from build123d import *

# Parameters (mm, degrees)
EXTRUDE_1_DEPTH          = 28.5
FILLET_3_R               = 4
CUT_EXTRUDE_1_DEPTH      = 31.686479107
CUT_EXTRUDE_1_DEPTH_BACK = 31.686479107
SKETCH_4_W               = 15
SKETCH_4_H               = 29
CUT_EXTRUDE_5_DEPTH      = 1.2
CUT_EXTRUDE_6_DEPTH      = 5
CUT_EXTRUDE_6_DEPTH_BACK = 25
SKETCH_5_R               = 2.6
CUT_EXTRUDE_7_DEPTH      = 31.823043328
DRAFT_1_ANGLE            = 60
SKETCH_7_W               = 10
SKETCH_7_H               = 1.2
SKETCH_7_H_2             = 0.5
CUT_EXTRUDE_8_DEPTH      = 31.686479107
DRAFT_3_ANGLE            = 30
SKETCH_8_W               = 17
SKETCH_8_H               = 30
CUT_EXTRUDE_9_DEPTH      = 2


with BuildPart() as part:
    # Эскиз2 → Бобышка-Вытянуть1 (new, symmetric)
    with BuildSketch(Plane.XY):
        Polygon((-10, 1.5), (-3, 2.9), (0, 2.9), (3, 2.9), (10, 1.5), (11, 1.5), (11, -1.5), (10, -1.5), (3, -2.9), (0, -2.9), (-3, -2.9), (-10, -1.5), (-11, -1.5), (-11, 1.5), align=None)
    extrude(amount=EXTRUDE_1_DEPTH, both=True)

    # Скругление3
    fillet_3_edges = [part.edges().sort_by_distance(p)[0] for p in [
        (-11, 0, -28.5),
        (-11, 0, 28.5),
        (11, 0, 28.5),
        (11, 0, -28.5),
    ]]
    fillet(fillet_3_edges, radius=FILLET_3_R)

    # Эскиз3 → Вырез-Вытянуть1 (cut, two sides: drawn at the far end of the back side and taken through both)
    with BuildSketch(Plane(origin=(0, 0, 0), x_dir=(0, 0, -1), z_dir=(1, 0, 0)).offset(-CUT_EXTRUDE_1_DEPTH_BACK)):
        Polygon((28.5, 2.9), (25.5, 2.9), (27.5, 1.5), (28.5, 1.5), align=None)
        Polygon((-27.5, -1.5), (-28.5, -1.5), (-28.5, -2.9), (-25.5, -2.9), align=None)
        Polygon((-25.5, 2.9), (-28.5, 2.9), (-28.5, 1.5), (-27.5, 1.5), align=None)
        Polygon((25.5, -2.9), (28.5, -2.9), (28.5, -1.5), (27.5, -1.5), align=None)
    extrude(amount=CUT_EXTRUDE_1_DEPTH + CUT_EXTRUDE_1_DEPTH_BACK, mode=Mode.SUBTRACT)

    # Эскиз4 → Вырез-Вытянуть5 (cut, symmetric)
    with BuildSketch(Plane(origin=(0, 0, 0), x_dir=(1, 0, 0), z_dir=(0, 1, 0))):
        with Locations((0, -12)):
            Rectangle(SKETCH_4_W, SKETCH_4_H)
    extrude(amount=CUT_EXTRUDE_5_DEPTH, both=True, mode=Mode.SUBTRACT)

    # Эскиз5 → Вырез-Вытянуть6 (cut, two sides: drawn at the far end of the back side and taken through both)
    with BuildSketch(Plane.XY.offset(-2.5).offset(-CUT_EXTRUDE_6_DEPTH_BACK)):
        with Locations(Location((0, 0, 0), (0, 0, 152.51357375))):
            Circle(SKETCH_5_R)
    extrude(amount=CUT_EXTRUDE_6_DEPTH + CUT_EXTRUDE_6_DEPTH_BACK, mode=Mode.SUBTRACT)

    # Эскиз6 → Вырез-Вытянуть7 (cut, through all)
    with BuildSketch(Plane.XZ.offset(-1.2)):
        Polygon((-2.306512519, -2.5), (2.306512519, -2.5), (7.5, -2.5), (7.5, 26.5), (-7.5, 26.5), (-7.5, -2.5), align=None)
    extrude(amount=-CUT_EXTRUDE_7_DEPTH, mode=Mode.SUBTRACT)

    # Уклон1
    draft_1_faces = [part.faces().sort_by_distance(p)[0] for p in [
        (0, -1.775343229, 2.5),
    ]]
    draft(draft_1_faces, Plane.ZX.offset(-1.2), DRAFT_1_ANGLE)

    # Эскиз7 → Вырез-Вытянуть8 (cut, through all)
    with BuildSketch(Plane(origin=(0, 0, 0), x_dir=(0, 0, -1), z_dir=(1, 0, 0))):
        with Locations((-13.5, -0.6)):
            Rectangle(SKETCH_7_W, SKETCH_7_H)
        with Locations((-13.5, -1.45)):
            Rectangle(SKETCH_7_W, SKETCH_7_H_2)
    extrude(amount=CUT_EXTRUDE_8_DEPTH, mode=Mode.SUBTRACT)

    # Уклон3
    draft_3_faces = [part.faces().sort_by_distance(p)[0] for p in [
        (0, -1.45, 13.5),
    ]]
    draft(draft_3_faces, Plane(origin=(11, 0, 18.5), x_dir=(-1, 0, 0), z_dir=(0, 0, -1)), DRAFT_3_ANGLE)

    # Эскиз8 → Вырез-Вытянуть9 (cut)
    with BuildSketch(Plane(origin=(0, 2.9, 0), x_dir=(1, 0, 0), z_dir=(0, 1, 0))):
        with Locations((0, -11.5)):
            Rectangle(SKETCH_8_W, SKETCH_8_H)
    extrude(amount=-CUT_EXTRUDE_9_DEPTH, mode=Mode.SUBTRACT)


solid = part.part
Work out the finished part from the listing and answer in its coordinate system (mm). A direction names the side the tool comes from. Round coordinates to 2 decimals unless told otherwise and drop trailing zeros. Write each loop counter-clockwise with the first axis right and the second up, starting at its lowest first coordinate (ties: lowest second). Pieces come first, ordered by that corner, then holes. Notation, with made-up numbers: (37.5, -2) -> (45.5, -2) arc R14 cw to (45.5, 4) -> close; hole circle Ø8 at (23.5, 52.5). An arc over 180 degrees is marked (long way). Write each question's results on one line, items separated by ' | '.
Item 1: Flat-ended cylindrical pins translate along their axes: P1, Ø0.5, axis at x = -4.5, z = -28, coming from the -Y side; P2, Ø1.1, axis at x = -1, z = -28, coming from the +Y side; P3, Ø1.8, axis at x = 9.5, z = 11.5, coming from the -Y side. Find the tip coordinate at first contact, or state that the pin passes through.
Result set:
P1: y = -1.5 | P2: y = 1.5 | P3: y = -1.78
Item 2: A cutting plane is placed at A-A, the plane z = -24. Determine the outline of the cut face in (x, y), plus the area to 3 significant figures.
Result set:
outline: (-11, -1.5) -> (-10, -1.5) -> (-3, -2.9) -> (3, -2.9) -> (10, -1.5) -> (11, -1.5) -> (11, 1.5) -> (10, 1.5) -> (3, 2.9) -> (-3, 2.9) -> (-10, 1.5) -> (-11, 1.5) -> close; hole circle Ø5.2 at (0, 0) | area: 81.2 mm^2
Item 3: Which of the six approach directions +Z, -Z, +X, -X, +Y, -Y give full straight-line access (tool end or side, diameter ignored) to faces 1 (the face through (-5, 0, -2.5)), 2 (the face through (6.6, -1.4, 18.5)), 3 (the face through (0, 0, -27.5))?
Result set:
face 1: +Y | face 2: +X | face 3: none
Item 4: Find the intervals of material crossed by line 1 along X through (y, z) = (0, -16); line 2 along Z through (x, y) = (-7.25, 0.3); line 3 along Y through (x, z) = (-0.25, -19), in increasing order. Write a range as [from, to].
Result set:
line 1: [-11, -2.6], [2.6, 11] | line 2: [-28.49, -2.5], [26.5, 28.49] | line 3: [-2.9, -2.59], [2.59, 2.9]
Item 5: A cutting plane is placed at B-B, the plane x = 1.25. Determine the outline of the cut face in (y, z), plus the area to 3 significant figures.
Result set:
outline: (-2.9, -25.5) -> (-2.28, -26.39) -> (-2.28, 0.63) -> (-1.2, 2.5) -> (-1.2, 8.5) -> (-1.7, 8.5) -> (-1.7, 18.5) -> (-1.2, 18.5) -> (-1.2, 26.5) -> (2.2, 26.5) -> (1.5, 27.5) -> (1.5, 28.5) -> (-1.5, 28.5) -> (-1.5, 27.5) -> (-2.9, 25.5) -> close; (-1.5, -28.5) -> (1.5, -28.5) -> (1.5, -27.5) -> (-1.5, -27.5) -> close; (2.28, -26.39) -> (2.9, -25.5) -> (2.9, -3.5) -> (2.28, -3.5) -> close | area: 77.7 mm^2
Item 6: The mould has two halves that part along Z. Classify faces 4 (the face through (7.5, 0.3, 11.8)), 5 (the face through (0, 0, -28.5)), 6 (the face through (0, -1.5, -28)): +Z half, -Z half, draft (parallel to the pull), parting line (faces both ways), or undercut.
Result set:
face 4: undercut | face 5: -Z half | face 6: draft
Item 7: A cutting plane is placed at D-D, the plane y = -0.65. Determine the outline of the cut face in (x, z).
Result set:
outline: (-11, -24.5) arc R4 ccw to (-7, -28.5) -> (7, -28.5) arc R4 ccw to (11, -24.5) -> (11, 8.5) -> (7.5, 8.5) -> (7.5, -2.5) -> (2.52, -2.5) -> (2.52, -27.5) -> (-2.52, -27.5) -> (-2.52, -2.5) -> (-7.5, -2.5) -> (-7.5, 26.5) -> (7.5, 26.5) -> (7.5, 18.5) -> (11, 18.5) -> (11, 24.5) arc R4 ccw to (7, 28.5) -> (-7, 28.5) arc R4 ccw to (-11, 24.5) -> close
Item 8: A cutting plane is placed at C-C, the plane x = 4.25. Determine the outline of the cut face in (y, z).
Result set:
outline: (-2.65, -25.86) -> (-1.5, -27.5) -> (-1.5, -28.5) -> (1.5, -28.5) -> (1.5, -27.5) -> (2.65, -25.86) -> (2.65, -3.5) -> (0.9, -3.5) -> (0.9, -2.5) -> (-1.2, -2.5) -> (-1.2, 8.5) -> (-1.7, 8.5) -> (-1.7, 18.5) -> (-1.2, 18.5) -> (-1.2, 26.5) -> (2.2, 26.5) -> (1.5, 27.5) -> (1.5, 28.5) -> (-1.5, 28.5) -> (-1.5, 27.5) -> (-2.65, 25.86) -> close
